For this review, take the finished solid that the model builds, in its own axes (mm). Face numbers are marked on the shaded views. Give positions to 0.01 mm unless a question says otherwise; leave off trailing zeros. Order: outer loops, then holes, each group sorted by start corner. A loop starts at its lowest first (then second) coordinate and runs counter-clockwise, first axis right, second up. Notation, with made-up numbers: (5, 49.5) - (11, 49.5) arc R25 cw to (11, 66.5) - close; hole circle Ø2 at (12.5, 76.25). An arc over 180 degrees is marked (long way). Use a Markdown table: item, result. Add a question column.
1) We need section B-B on z = 1.45. Write out the cut boundary in (x, y), then the cut area to 3 significant figures.
2) We need section A-A on x = 0. Write out the cut boundary in (y, z).
3) Mouldability with a two-part tool opening along Y and no side actions: class the marked faces 1, 2 and 3 as released by +Y, released by -Y, zero draft, split by the parting line, or undercut.
4) Wall thickness on L1, parallel to Y at x = 0, z = 1.45; L2, parallel to X at y = 0.75, z = 1.1: over which ranges is each line inside the solid? List them lowest first.
5) Clearance check with a flat-ended pin moving along its axis: P1, Ø2.5, axis at x = 0, y = 0, coming from the -Z side. State where the tip first meets the part, or that it passes through.
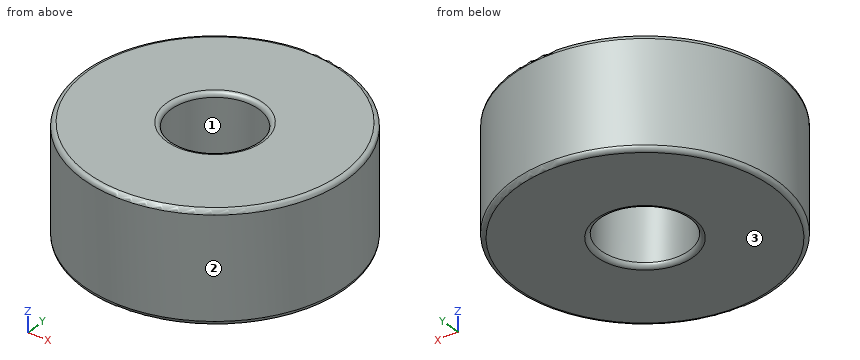
```python
from build123d import *

# Parameters (mm, degrees)
SKETCH1_R           = 3
SKETCH1_R_2         = 1
BOSS_EXTRUDE1_DEPTH = 2.5
FILLET1_R           = 0.1
FILLET2_R           = 0.1


with BuildPart() as part:
    # Sketch1 → Boss-Extrude1 (new body)
    with BuildSketch(Plane.XY):
        Circle(SKETCH1_R)
        Circle(SKETCH1_R_2, mode=Mode.SUBTRACT)
    extrude(amount=BOSS_EXTRUDE1_DEPTH)

    # Fillet1
    fillet1_edges = [part.edges().sort_by_distance(p)[0] for p in [
        (-3, 0, 2.5),
    ]]
    fillet(fillet1_edges, radius=FILLET1_R)

    # Fillet2
    fillet2_edges = [part.edges().sort_by_distance(p)[0] for p in [
        (-3, 0, 0),
        (-1, 0, 0),
        (-1, 0, 2.5),
    ]]
    fillet(fillet2_edges, radius=FILLET2_R)


solid = part.part
```
Checked values:
| question | item | result |
|---|---|---|
| 1 | outline | circle Ø6 at (0, 0); hole circle Ø2 at (0, 0) |
| 1 | area | 25.1 mm² |
| 2 | outline | (-3, 0.1) arc R0.1 ccw to (-2.9, 0) - (-1.1, 0) arc R0.1 ccw to (-1, 0.1) - (-1, 2.4) arc R0.1 ccw to (-1.1, 2.5) - (-2.9, 2.5) arc R0.1 ccw to (-3, 2.4) - close; (1, 0.1) arc R0.1 ccw to (1.1, 0) - (2.9, 0) arc R0.1 ccw to (3, 0.1) - (3, 2.4) arc R0.1 ccw to (2.9, 2.5) - (1.1, 2.5) arc R0.1 ccw to (1, 2.4) - close |
| 3 | face 1 | undercut |
| 3 | face 2 | split by the parting line |
| 3 | face 3 | zero draft |
| 4 | L1 | -3 to -1, 1 to 3 |
| 4 | L2 | -2.9 to -0.66, 0.66 to 2.9 |
| 5 | P1 | z = 0 |
